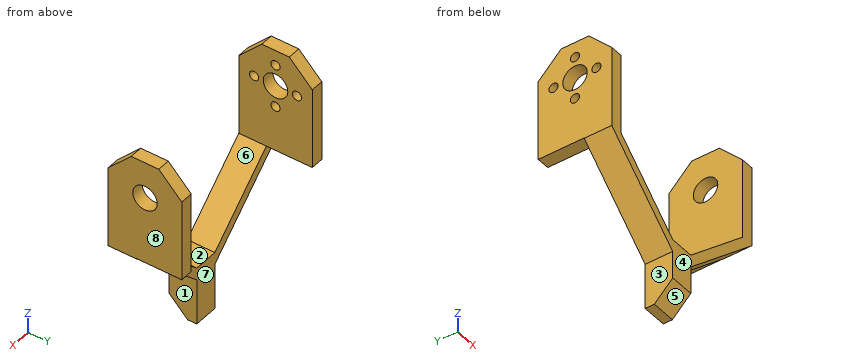
from build123d import *

# Parameters (mm, degrees)
BOSS_EXTRUDE1_DEPTH = 62
CUT_EXTRUDE1_REACH  = 83.419
BOSS_EXTRUDE2_START = -15
SKETCH9_W           = 8
SKETCH9_H           = 15
BOSS_EXTRUDE2_DEPTH = 9
SKETCH7_R           = 4
CUT_EXTRUDE4_DEPTH  = 70
CUT_EXTRUDE5_REACH  = 90.499
SKETCH8_R           = 1.5
CHAMFER1_SIZE       = 7.5
CUT_EXTRUDE6_DEPTH  = 15
CHAMFER2_SIZE       = 6


with BuildPart() as part:
    # Sketch1 → Boss-Extrude1 (new body)
    with BuildSketch(Plane(origin=(0, 0, 0), x_dir=(0, 0, -1), z_dir=(1, 0, 0))):
        Polygon((-12, 12), (-12, -12), (12, -12), (47, -12), (47, 12), (12, 12), align=None)
    extrude(amount=-BOSS_EXTRUDE1_DEPTH)

    # Sketch2 → Cut-Extrude1 (cut, up to next)
    with BuildSketch(Plane(origin=(0, 12, 0), x_dir=(1, 0, 0), z_dir=(0, 1, 0)), mode=Mode.PRIVATE) as cut_extrude1_sk1:
        Polygon((-57.8, -12), (-57.8, 21.888888889), (-35, 43), (-27, 43), (-4.2, 21.888888889), (-4.2, -12), align=None)
    cut_extrude1_tool1 = extrude(cut_extrude1_sk1.sketch, amount=-CUT_EXTRUDE1_REACH, mode=Mode.PRIVATE) & part.part
    # Sketch2 → Cut-Extrude1 (cut, up to next)
    with BuildSketch(Plane(origin=(0, 12, 0), x_dir=(1, 0, 0), z_dir=(0, 1, 0)), mode=Mode.PRIVATE) as cut_extrude1_sk2:
        Polygon((-62, 22), (-62, 47), (-35, 47), align=None)
    cut_extrude1_tool2 = extrude(cut_extrude1_sk2.sketch, amount=-CUT_EXTRUDE1_REACH, mode=Mode.PRIVATE) & part.part
    # Sketch2 → Cut-Extrude1 (cut, up to next)
    with BuildSketch(Plane(origin=(0, 12, 0), x_dir=(1, 0, 0), z_dir=(0, 1, 0)), mode=Mode.PRIVATE) as cut_extrude1_sk3:
        Polygon((-27, 47), (0, 47), (0, 22), align=None)
    cut_extrude1_tool3 = extrude(cut_extrude1_sk3.sketch, amount=-CUT_EXTRUDE1_REACH, mode=Mode.PRIVATE) & part.part
    add(cut_extrude1_tool1.solids().sort_by_distance((-31, 12, -11.506957))[0], mode=Mode.SUBTRACT)
    add(cut_extrude1_tool2.solids().sort_by_distance((-53, 12, -38.666667))[0], mode=Mode.SUBTRACT)
    add(cut_extrude1_tool3.solids().sort_by_distance((-9, 12, -38.666667))[0], mode=Mode.SUBTRACT)

    # Sketch9 → Boss-Extrude2 (add)
    with BuildSketch(Plane(origin=(0, 12, 0), x_dir=(1, 0, 0), z_dir=(0, 1, 0)).offset(BOSS_EXTRUDE2_START)):
        with Locations((-31, 54.5)):
            Rectangle(SKETCH9_W, SKETCH9_H)
    extrude(amount=-BOSS_EXTRUDE2_DEPTH)

    # Sketch7 → Cut-Extrude4 (cut)
    with BuildSketch(Plane(origin=(0, 0, 0), x_dir=(0, 0, -1), z_dir=(1, 0, 0))):
        Circle(SKETCH7_R)
    extrude(amount=-CUT_EXTRUDE4_DEPTH, mode=Mode.SUBTRACT)

    # Sketch8 → Cut-Extrude5 (cut, up to next)
    with BuildSketch(Plane.ZY.offset(62), mode=Mode.PRIVATE) as cut_extrude5_sk1:
        with Locations((0, 7)):
            Circle(SKETCH8_R)
    cut_extrude5_tool1 = extrude(cut_extrude5_sk1.sketch, amount=-CUT_EXTRUDE5_REACH, mode=Mode.PRIVATE) & part.part
    # Sketch8 → Cut-Extrude5 (cut, up to next)
    with BuildSketch(Plane.ZY.offset(62), mode=Mode.PRIVATE) as cut_extrude5_sk2:
        with Locations((7, 0)):
            Circle(SKETCH8_R)
    cut_extrude5_tool2 = extrude(cut_extrude5_sk2.sketch, amount=-CUT_EXTRUDE5_REACH, mode=Mode.PRIVATE) & part.part
    # Sketch8 → Cut-Extrude5 (cut, up to next)
    with BuildSketch(Plane.ZY.offset(62), mode=Mode.PRIVATE) as cut_extrude5_sk3:
        with Locations((0, -7)):
            Circle(SKETCH8_R)
    cut_extrude5_tool3 = extrude(cut_extrude5_sk3.sketch, amount=-CUT_EXTRUDE5_REACH, mode=Mode.PRIVATE) & part.part
    # Sketch8 → Cut-Extrude5 (cut, up to next)
    with BuildSketch(Plane.ZY.offset(62), mode=Mode.PRIVATE) as cut_extrude5_sk4:
        with Locations((-7, 0)):
            Circle(SKETCH8_R)
    cut_extrude5_tool4 = extrude(cut_extrude5_sk4.sketch, amount=-CUT_EXTRUDE5_REACH, mode=Mode.PRIVATE) & part.part
    add(cut_extrude5_tool1.solids().sort_by_distance((-62, 7, 0))[0], mode=Mode.SUBTRACT)
    add(cut_extrude5_tool2.solids().sort_by_distance((-62, 0, 7))[0], mode=Mode.SUBTRACT)
    add(cut_extrude5_tool3.solids().sort_by_distance((-62, -7, 0))[0], mode=Mode.SUBTRACT)
    add(cut_extrude5_tool4.solids().sort_by_distance((-62, 0, -7))[0], mode=Mode.SUBTRACT)

    # Chamfer1
    chamfer1_edges = [part.edges().sort_by_distance(p)[0] for p in [
        (-59.9, -12, 12),
        (-59.9, 12, 12),
        (-2.1, 12, 12),
        (-2.1, -12, 12),
    ]]
    chamfer(chamfer1_edges, length=CHAMFER1_SIZE)

    # Sketch10 → Cut-Extrude6 (cut)
    with BuildSketch(Plane(origin=(0, 12, 0), x_dir=(1, 0, 0), z_dir=(0, 1, 0))):
        Polygon((-62, 22), (-35, 47), (-27, 47), (0, 22), (0, 21.888888889), (-4.2, 21.888888889), (-27, 43), (-35, 43), (-57.8, 21.888888889), (-62, 21.888888889), align=None)
    extrude(amount=-CUT_EXTRUDE6_DEPTH, mode=Mode.SUBTRACT)

    # Chamfer2
    chamfer2_edges = [part.edges().sort_by_distance(p)[0] for p in [
        (-31, -12, -62),
    ]]
    chamfer(chamfer2_edges, length=CHAMFER2_SIZE)


solid = part.part
Could you check a few things on this model? Use its own coordinates, in mm. Face numbers are marked on the shaded views. A direction names the side the tool comes from. Give positions to 0.01 mm unless a question says otherwise; leave off trailing zeros. Write each loop counter-clockwise with the first axis right and the second up, starting at its lowest first coordinate (ties: lowest second). Pieces come first, ordered by that corner, then holes. Notation, with made-up numbers: (30, -34.5) -> (64, -34.5) arc R11 cw to (64, -30.5) -> close; hole circle Ø1 at (40.25, 73.25). An arc over 180 degrees is marked (long way). Answer as CSV lines item,"result". Start each with the question number.
(1) Please list where these lines run through material, in increasing order: line 1 (Y direction, x = -61.05, z = 0); line 2 (Y direction, x = -2.7, z = 0); line 3 (X direction, y = 10.25, z = -18.5).
(2) If we section it at D-D, the plane y = -7: Write out the boundary of the cut face in (x, z), and give its area (3 significant figures).
(3) If we section it at B-B, the plane z = -36: Write out the boundary of the cut face in (x, y).
(4) If we mould it in two halves opening along X, with no side actions, what happens to the marked faces 6, 7 and 8? For each: +X half, -X half, draft (parallel to the pull), parting line (faces both ways), or undercut.
(5) Which directions (+Z, -Z, +X, -X, +Y, -Y) give clear straight access to the entire face, cutting with the end or side of a thin tool? Please do the marked faces 1, 2, 3, 4 and 5.
(6) If we section it at A-A, the plane z = -7: Write out the boundary of the cut face in (x, y), and give its area (3 significant figures).
(7) I'm going to push flat-ended pins straight in: pin 1 Ø10 at (x, z) = (-17, -25.5) entering from +Y; pin 2 Ø2 at (x, y) = (-60, 6.5) entering from -Z; pin 3 Ø5 at (x, y) = (-23.5, -7.5) entering from +Z; pin 4 Ø2.5 at (y, z) = (-7, -54) entering from +X. Where does each tip first touch, or does it pass through?
(8) If we section it at C-C, the plane y = 7: Write out the boundary of the cut face in (x, z).
Answer list:
1,line 1,"-12 to -8.5, -5.5 to -4, 4 to 5.5, 8.5 to 12"
1,line 2,"-12 to -4, 4 to 12"
1,line 3,"-62 to -57.8, -4.2 to 0"
2,outline,"(-62, -22) -> (-35, -47) -> (-35, -61) -> (-27, -61) -> (-27, -47) -> (0, -22) -> (0, 9.5) -> (-4.2, 9.5) -> (-4.2, -21.89) -> (-27, -43) -> (-35, -43) -> (-57.8, -21.89) -> (-57.8, -1.5) -> (-62, -1.5) -> close; (-62, 1.5) -> (-57.8, 1.5) -> (-57.8, 9.5) -> (-62, 9.5) -> close"
2,area,"595 mm^2"
3,outline,"(-46.88, -12) -> (-42.56, -12) -> (-42.56, -3) -> (-46.88, -3) -> close; (-19.44, -12) -> (-15.12, -12) -> (-15.12, -3) -> (-19.44, -3) -> close"
4,face 6,"undercut"
4,face 7,"draft"
4,face 8,"+X half"
5,face 1,"-Z, +X, +Y, -Y"
5,face 2,"+Z, +Y, -Y"
5,face 3,"-Z, -X, +Y, -Y"
5,face 4,"+Z, -Z, +X, -X, -Y"
5,face 5,"-Z, +X, -X, -Y"
6,outline,"(-62, -12) -> (-57.8, -12) -> (-57.8, -1.5) -> (-62, -1.5) -> close; (-62, 1.5) -> (-57.8, 1.5) -> (-57.8, 12) -> (-62, 12) -> close; (-4.2, -12) -> (0, -12) -> (0, 12) -> (-4.2, 12) -> close"
6,area,"189 mm^2"
7,pin 1,"through"
7,pin 2,"z = -21.89"
7,pin 3,"z = -37.44"
7,pin 4,"x = -27"
8,outline,"(-62, -21.89) -> (-57.8, -21.89) -> (-57.8, -1.5) -> (-62, -1.5) -> close; (-62, 1.5) -> (-57.8, 1.5) -> (-57.8, 9.5) -> (-62, 9.5) -> close; (-4.2, -21.89) -> (0, -21.89) -> (0, 9.5) -> (-4.2, 9.5) -> close"
